from build123d import *

# Parameters (mm, degrees)
F1_DEPTH = 5
F3_DEPTH = 1


with BuildPart() as f1:
    # F0 (on Front) → F1 (new body)
    with BuildSketch(Plane.XZ):
        Polygon((0, 6.928203), (-6, 3.464102), (-6, -3.464102), (0, -6.928203), (6, -3.464102), (6, 3.464102), align=None)
        Polygon((0, -5.773503), (-5, -2.886751), (-5, 2.886751), (0, 5.773503), (5, 2.886751), (5, -2.886751), align=None, mode=Mode.SUBTRACT)
    extrude(amount=-F1_DEPTH)

    # F2 (on face) → F3 (join)
    with BuildSketch(Plane(origin=(0, 5, 0), x_dir=(-1, 0, 0), z_dir=(0, 1, 0))):
        Polygon((6, 3.464102), (0, 6.928203), (-6, 3.464102), (-6, -3.464102), (0, -6.928203), (6, -3.464102), align=None)
    extrude(amount=-F3_DEPTH)


solid = f1.part
Design review of the part built by this model. Coordinates are the model's own, in mm. A direction names the side the tool comes from. Round coordinates to 2 decimals unless told otherwise and drop trailing zeros. Loops run counter-clockwise (first coordinate to the right, second up) from the corner with the lowest first, then second, coordinate; pieces in that order, holes last. Notation, with made-up numbers: (57.25, 9) -> (85.25, 9) arc R12 ccw to (85.25, 23) -> close; hole circle Ø1 at (37.25, 49). An arc over 180 degrees is marked (long way). Use one line per item in the form item = value. Start each with the question number.
Q1. For pin 1 Ø3 at (x, z) = (-1, 1) entering from -Y; pin 2 Ø2 at (x, y) = (-3.5, 2.5) entering from -Z, all flat-tipped, find the tip position at first contact; note any pin that passes through.
Q2. Wall thickness on line 1 along X through (y, z) = (0.35, 2); line 2 along Y through (x, z) = (3, -3.5); line 3 along Z through (x, y) = (4.75, 0.4): over which ranges is each line inside the solid? List them lowest first. Write a range as [from, to].
Q3. We need section B-B on x = -0.5. Give the boundary of the cut face in (y, z), then the cut area to 3 significant figures.
Q4. Machinability: for faces 1 (the face through (-6, 2, 0)), 2 (the face through (-5, 2, 0)), which of the approach directions +Z, -Z, +X, -X, +Y, -Y give a long, thin tool a straight path to every point of the face, cutting with its end or side? Answer none if there is none.
Q5. We need section C-C on y = 4.75. Give the boundary of the cut face in (x, z), then the cut area to 3 significant figures.
Q6. We need section D-D on z = -4. Give the boundary of the cut face in (x, y), then the cut area to 3 significant figures.
Q7. We need section A-A on y = 0.45. Give the boundary of the cut face in (x, z), then the cut area to 3 significant figures.
Q8. Draft analysis for pull direction Z (two halves, no side actions). For faces 3 (the face through (2.96, 2.46, -5.22)), 4 (the face through (2, 0, -5)), 5 (the face through (2.535, 1.972, -4.31)), state which applies: +Z half, -Z half, draft (parallel to the pull), parting line (faces both ways), or undercut.
Calculated:
q1.pin_1 = 4
q1.pin_2 = -5.48
q2.line_1 = [-6, -5], [5, 6]
q2.line_2 = [4, 5]
q2.line_3 = [-4.19, -3.03], [3.03, 4.19]
q3.outline = (0, -6.64) -> (5, -6.64) -> (5, 6.64) -> (0, 6.64) -> (0, 5.48) -> (4, 5.48) -> (4, -5.48) -> (0, -5.48) -> close
q3.area = 22.5 mm²
q4.face_1 = +Z, -Z, -X, +Y, -Y
q4.face_2 = -Y
q5.outline = (-6, -3.46) -> (0, -6.93) -> (6, -3.46) -> (6, 3.46) -> (0, 6.93) -> (-6, 3.46) -> close
q5.area = 125 mm²
q6.outline = (-5.07, 0) -> (-3.07, 0) -> (-3.07, 4) -> (3.07, 4) -> (3.07, 0) -> (5.07, 0) -> (5.07, 5) -> (-5.07, 5) -> close
q6.area = 26.1 mm²
q7.outline = (-6, -3.46) -> (0, -6.93) -> (6, -3.46) -> (6, 3.46) -> (0, 6.93) -> (-6, 3.46) -> close; hole (-5, -2.89) -> (0, -5.77) -> (5, -2.89) -> (5, 2.89) -> (0, 5.77) -> (-5, 2.89) -> close
q7.area = 38.1 mm²
q8.face_3 = -Z half
q8.face_4 = draft
q8.face_5 = undercut
